from build123d import *

# Parameters (mm, degrees)
SKETCH_W        = 160
SKETCH_H        = 70
PAD_DEPTH       = 10
SKETCH001_R     = 10
POCKET_DEPTH    = 10
SKETCH002_R     = 8
PAD001_DEPTH    = 10
SKETCH003_R     = 4.2
POCKET001_DEPTH = 20
SKETCH004_W     = 50
SKETCH004_H     = 50
SKETCH004_W_2   = 39.2
SKETCH004_H_2   = 39.2
PAD002_DEPTH    = 5
SKETCH005_R     = 1.6
POCKET002_DEPTH = 10
SKETCH006_R     = 4.2
POCKET003_DEPTH = 10
SKETCH007_W     = 25
SKETCH007_H     = 20
PAD003_DEPTH    = 40
SKETCH008_W     = 8
SKETCH008_H     = 20
POCKET004_DEPTH = 30
SKETCH009_W     = 13.2
SKETCH009_H     = 11.2
POCKET005_DEPTH = 20
SKETCH010_W     = 8.5
SKETCH010_H     = 12
PAD004_DEPTH    = 5
SKETCH011_R     = 1.5
POCKET006_DEPTH = 25
CHAMFER_SIZE    = 4.95
CHAMFER001_SIZE = 4.95
CHAMFER002_SIZE = 4.95
CHAMFER003_SIZE = 4.95
FILLET_R        = 20
FILLET001_R     = 20
FILLET002_R     = 20
FILLET003_R     = 20
SKETCH012_W     = 8
SKETCH012_H     = 10
PAD005_DEPTH    = 8.5
SKETCH013_W     = 8
SKETCH013_H     = 10
PAD006_DEPTH    = 8.5
CHAMFER004_SIZE = 7
CHAMFER005_SIZE = 7


with BuildPart() as part:
    # Sketch → Pad (new body)
    with BuildSketch(Plane.XY):
        Rectangle(SKETCH_W, SKETCH_H)
    extrude(amount=PAD_DEPTH)

    # Sketch001 (on Face6 of Pad) → Pocket (cut)
    with BuildSketch(Plane.XY.offset(10)):
        Circle(SKETCH001_R)
    extrude(amount=-POCKET_DEPTH, mode=Mode.SUBTRACT)

    # Sketch002 (on Face5 of Pocket) → Pad001 (join)
    with BuildSketch(Plane.XY.offset(10)):
        with Locations((-40, 0)):
            Circle(SKETCH002_R)
        with Locations((40, 0)):
            Circle(SKETCH002_R)
    extrude(amount=PAD001_DEPTH)

    # Sketch003 (on Face10 of Pad001) → Pocket001 (cut)
    with BuildSketch(Plane.XY.offset(20)):
        with Locations((-40, 0)):
            Circle(SKETCH003_R)
        with Locations((40, 0)):
            Circle(SKETCH003_R)
    extrude(amount=-POCKET001_DEPTH, mode=Mode.SUBTRACT)

    # Sketch004 (on Face5 of Pocket001) → Pad002 (join)
    with BuildSketch(Plane.XY.offset(10)):
        Rectangle(SKETCH004_W, SKETCH004_H)
        Rectangle(SKETCH004_W_2, SKETCH004_H_2, mode=Mode.SUBTRACT)
    extrude(amount=PAD002_DEPTH)

    # Sketch005 (on Face17 of Pad002) → Pocket002 (cut)
    with BuildSketch(Plane.XY.offset(10)):
        with Locations((-15.5, 15.5)):
            Circle(SKETCH005_R)
        with Locations((15.5, 15.5)):
            Circle(SKETCH005_R)
        with Locations((-15.5, -15.5)):
            Circle(SKETCH005_R)
        with Locations((15.5, -15.5)):
            Circle(SKETCH005_R)
    extrude(amount=-POCKET002_DEPTH, mode=Mode.SUBTRACT)

    # Sketch006 (on Face5 of Pocket002) → Pocket003 (cut)
    with BuildSketch(Plane.XY.offset(10)):
        with Locations((-60, 0)):
            Circle(SKETCH006_R)
        with Locations((60, 0)):
            Circle(SKETCH006_R)
    extrude(amount=-POCKET003_DEPTH, mode=Mode.SUBTRACT)

    # Sketch007 (on Face4 of Pocket003) → Pad003 (join)
    with BuildSketch(Plane(origin=(0, 0, 0), x_dir=(1, 0, 0), z_dir=(0, 0, -1))):
        with Locations((0, 45)):
            Rectangle(SKETCH007_W, SKETCH007_H)
    extrude(amount=-PAD003_DEPTH)

    # Sketch008 (on Face31 of Pad003) → Pocket004 (cut)
    with BuildSketch(Plane.XY.offset(40)):
        with Locations((0, -45)):
            Rectangle(SKETCH008_W, SKETCH008_H)
    extrude(amount=-POCKET004_DEPTH, mode=Mode.SUBTRACT)

    # Sketch009 (on Face33 of Pocket004) → Pocket005 (cut)
    with BuildSketch(Plane.XY.offset(40)):
        with Locations((0, -44.7)):
            Rectangle(SKETCH009_W, SKETCH009_H)
    extrude(amount=-POCKET005_DEPTH, mode=Mode.SUBTRACT)

    # Sketch010 (on Face29 of Pocket005) → Pad004 (join)
    with BuildSketch(Plane.XZ.offset(55)):
        with Locations((-8.25, 34)):
            Rectangle(SKETCH010_W, SKETCH010_H)
        with Locations((8.25, 34)):
            Rectangle(SKETCH010_W, SKETCH010_H)
    extrude(amount=PAD004_DEPTH)

    # Sketch011 (on Face28 of Pad004) → Pocket006 (cut)
    with BuildSketch(Plane.YZ.offset(12.5)):
        with Locations((-56, 34)):
            Circle(SKETCH011_R)
    extrude(amount=-POCKET006_DEPTH, mode=Mode.SUBTRACT)

    # Chamfer
    chamfer_edges = [part.edges().sort_by_distance(p)[0] for p in [
        (8.25, -60, 28),
    ]]
    chamfer(chamfer_edges, length=CHAMFER_SIZE)

    # Chamfer001
    chamfer001_edges = [part.edges().sort_by_distance(p)[0] for p in [
        (-8.25, -60, 28),
    ]]
    chamfer(chamfer001_edges, length=CHAMFER001_SIZE)

    # Chamfer002
    chamfer002_edges = [part.edges().sort_by_distance(p)[0] for p in [
        (8.25, -60, 40),
    ]]
    chamfer(chamfer002_edges, length=CHAMFER002_SIZE)

    # Chamfer003
    chamfer003_edges = [part.edges().sort_by_distance(p)[0] for p in [
        (-8.25, -60, 40),
    ]]
    chamfer(chamfer003_edges, length=CHAMFER003_SIZE)

    # Fillet
    fillet_edges = [part.edges().sort_by_distance(p)[0] for p in [
        (-80, -35, 5),
    ]]
    fillet(fillet_edges, radius=FILLET_R)

    # Fillet001
    fillet001_edges = [part.edges().sort_by_distance(p)[0] for p in [
        (-80, 35, 5),
    ]]
    fillet(fillet001_edges, radius=FILLET001_R)

    # Fillet002
    fillet002_edges = [part.edges().sort_by_distance(p)[0] for p in [
        (80, -35, 5),
    ]]
    fillet(fillet002_edges, radius=FILLET002_R)

    # Fillet003
    fillet003_edges = [part.edges().sort_by_distance(p)[0] for p in [
        (80, 35, 5),
    ]]
    fillet(fillet003_edges, radius=FILLET003_R)

    # Sketch012 (on Face22 of Fillet003) → Pad005 (join)
    with BuildSketch(Plane.YZ.offset(12.5)):
        with Locations((-31, 15)):
            Rectangle(SKETCH012_W, SKETCH012_H)
    extrude(amount=-PAD005_DEPTH)

    # Sketch013 (on Face24 of Pad005) → Pad006 (join)
    with BuildSketch(Plane(origin=(-12.5, 0, 0), x_dir=(0, -1, 0), z_dir=(-1, 0, 0))):
        with Locations((31, 15)):
            Rectangle(SKETCH013_W, SKETCH013_H)
    extrude(amount=-PAD006_DEPTH)

    # Chamfer004
    chamfer004_edges = [part.edges().sort_by_distance(p)[0] for p in [
        (8.25, -27, 20),
    ]]
    chamfer(chamfer004_edges, length=CHAMFER004_SIZE)

    # Chamfer005
    chamfer005_edges = [part.edges().sort_by_distance(p)[0] for p in [
        (-8.25, -27, 20),
    ]]
    chamfer(chamfer005_edges, length=CHAMFER005_SIZE)


solid = part.part
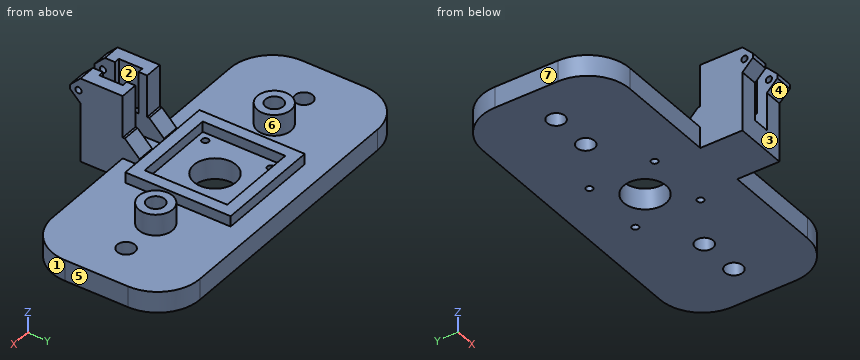
Design review of the part built by this model. Coordinates are the model's own, in mm. Face numbers are marked on the shaded views. A direction names the side the tool comes from. Coordinates: 2 decimals unless noted, no trailing zeros. Write each loop counter-clockwise with the first axis right and the second up, starting at its lowest first coordinate (ties: lowest second). Pieces come first, ordered by that corner, then holes. Notation, with made-up numbers: (61.5, 81.25) -> (74.5, 81.25) arc R29 cw to (74.5, 104.25) -> close; hole circle Ø5 at (18, -3). An arc over 180 degrees is marked (long way). Write each question's results on one line, items separated by ' | '. Start each with the question number.
(1) Take a section at A-A on z = 23. Write out the cut boundary in (x, y).
(2) Take a section at B-B on x = 0. Write out the cut boundary in (y, z).
(3) For line 1 along Y through (x, z) = (-15.5, 6); line 2 along Y through (x, z) = (-15, 6); line 3 along X through (y, z) = (-48, 22), list the stretches that pass through material, from the lowest coordinate up. Write a range as from..to.
(4) Clearance check with flat-ended pins moving along their axes: P1, Ø2, axis at x = -5, y = -42, coming from the +Z side; P2, Ø12.5, axis at x = -5, z = 18.5, coming from the -Y side; P3, Ø0.8, axis at x = 5, z = 29.5, coming from the +Y side. State where each tip first meets the part, or that it passes through.
(5) The part is to be moulded in two halves that separate along X. For the marked faces 4, 5, 6 and 7, say which applies: pulls with the +X half, pulls with the -X half, needs draft (parallel to the pull), parting line crosses it, or undercut.
(6) Take a section at C-C on y = 0. Give the number of separate pieces and of enclosed holes in the cut face, and give its area (3 significant figures).
(7) Take a section at D-D on x = -40. Write out the cut boundary in (y, z).
(8) Tool access review of the marked faces 1, 2 and 3: name each direction out of +Z, -Z, +X, -X, +Y, -Y from which nothing blocks a thin tool from reaching the whole face with its end or side.
Results found:
1) outline: (-12.5, -55) -> (-4, -55) -> (-4, -50.3) -> (-6.6, -50.3) -> (-6.6, -39.1) -> (-4, -39.1) -> (-4, -35) -> (-12.5, -35) -> close; (4, -55) -> (12.5, -55) -> (12.5, -35) -> (4, -35) -> (4, -39.1) -> (6.6, -39.1) -> (6.6, -50.3) -> (4, -50.3) -> close
2) outline: (-55, 0) -> (-10, 0) -> (-10, 10) -> (-19.6, 10) -> (-19.6, 15) -> (-25, 15) -> (-25, 10) -> (-55, 10) -> close; (10, 0) -> (35, 0) -> (35, 10) -> (25, 10) -> (25, 15) -> (19.6, 15) -> (19.6, 10) -> (10, 10) -> close
3) line 1: y = -35..-17.1, -13.9..13.9, 17.1..35 | line 2: y = -35..-17.02, -13.98..13.98, 17.02..35 | line 3: x = -12.5..-6.6, 6.6..12.5
4) P1: stops at z = 20 | P2: stops at y = -55 | P3: stops at y = -35
5) face 4: needs draft | face 5: pulls with the +X half | face 6: undercut | face 7: pulls with the -X half
6) separate pieces: 6 | enclosed holes: 0 | area: 1,270 mm2
7) outline: (-35, 0) -> (-4.2, 0) -> (-4.2, 20) -> (-8, 20) -> (-8, 10) -> (-35, 10) -> close; (4.2, 0) -> (35, 0) -> (35, 10) -> (8, 10) -> (8, 20) -> (4.2, 20) -> close
8) face 1: +Z, -Z, +X, -Y | face 2: +Z | face 3: -Z, +X, -X, -Y
